Read the model definition and answer for the solid it produces. Units are mm, in the model's axes. Face numbers are marked on the shaded views. A direction names the side the tool comes from. Coordinates: 2 decimals unless noted, no trailing zeros. Loops run counter-clockwise (first coordinate to the right, second up) from the corner with the lowest first, then second, coordinate; pieces in that order, holes last. Notation, with made-up numbers: M -9,41 L 29,41 A16 ccw 29,65 Z; hole C 18,86.5 d2. An arc over 180 degrees is marked long. Use one line per item in the form item = value. Start each with the question number.
1. The part is cut by section A-A (x = 20.5). Give the vertices of the cut face in (y, z), plus the area to 3 significant figures.
2. The part is cut by section C-C (z = 12.5). Give the vertices of the cut face in (x, y).
3. A tool of negligible diameter and unlimited length cuts with its end or side. For the marked faces 4, 5 and 6, from which of +Z, -Z, +X, -X, +Y, -Y can it reach the whole face along a straight path? Write none if from no direction.
4. Flat-ended cylindrical pins translate along their axes: pin 1 (3 mm diameter, centred on y = 37, z = -24.5, fed in from +X); pin 2 (3 mm diameter, centred on x = 13.5, z = 20.5, fed in from +Y); pin 3 (12 mm diameter, centred on x = 12.5, z = 16, fed in from +Y); pin 4 (10 mm diameter, centred on y = -0.5, z = 29.5, fed in from -X). Find the tip coordinate at first contact, or state that the pin passes through.
5. For a pull along Y with two mould halves and no side action, classify the marked faces 1, 2 and 3 as released by +Y, released by -Y, zero draft, split by the parting line, or undercut.
6. The part is cut by section D-D (x = 28). Give the vertices of the cut face in (y, z), plus the area to 3 significant figures.
7. Find the intervals of material crossed by probe 1 along Y at (x, z) = (8, -8.5); probe 2 along Y at (x, z) = (28, 6); probe 3 along X at (y, z) = (-36, -13), in increasing order. Write a range as [from, to].
8. The part is cut by section B-B (y = 0). Give the vertices of the cut face in (x, z).
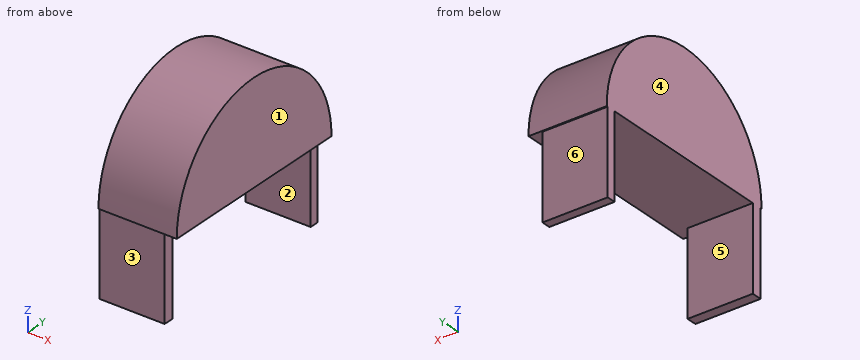
from build123d import *

# Parameters (mm, degrees)
F1_DEPTH = 5.08
F2_DEPTH = 25.4
F3_W     = 3.4888088703
F3_H     = 32.5622074306
F3_W_2   = 3.9539821446
F4_DEPTH = 25.4


with BuildPart() as f1:
    # F0 (on Right) → F1 (new body)
    with BuildSketch(Plane.YZ):
        with BuildLine():
            Line((-39.5398288965, 0), (39.5398288965, 0))
            ThreePointArc((39.5398288965, 0), (0, 39.5398288965), (-39.5398288965, 0))
        make_face()
    extrude(amount=F1_DEPTH)

    # F2 (add): a face of the model
    f2_faces = [f1.faces().sort_by_distance(p)[0] for p in [
        (5.08, 0, 16.781224581),
    ]]
    extrude(f2_faces, amount=F2_DEPTH)

    # F3 (on Right) → F4 (join)
    with BuildSketch(Plane.YZ):
        with Locations((37.3302474618, -16.2811037153)):
            Rectangle(F3_W, F3_H)
        with Locations((-37.0976608247, -16.2811037153)):
            Rectangle(F3_W_2, F3_H)
    extrude(amount=F4_DEPTH)


solid = f1.part
Computed values:
q1.outline = M -39.54,0 L -39.07,0 L -39.07,-32.56 L -35.12,-32.56 L -35.12,0 L 35.59,0 L 35.59,-32.56 L 39.07,-32.56 L 39.07,0 L 39.54,0 A39.54 ccw Z
q1.area = 2,700 mm²
q2.outline = M 0,-37.51 L 30.48,-37.51 L 30.48,37.51 L 0,37.51 Z
q3.face_4 = +Z, -Z, -X, +Y, -Y
q3.face_5 = -Z, +X, -X
q3.face_6 = -Z, +X, -X, +Y
q4.pin_1 = 25.4
q4.pin_2 = 34.68
q4.pin_3 = 38.25
q4.pin_4 = 0
q5.face_1 = zero draft
q5.face_2 = undercut
q5.face_3 = released by -Y
q6.outline = M -39.54,0 L 39.54,0 A39.54 ccw Z
q6.area = 2,460 mm²
q7.probe_1 = [-39.07, -35.12], [35.59, 39.07]
q7.probe_2 = [-39.08, 39.08]
q7.probe_3 = [0, 25.4]
q8.outline = M 0,0 L 30.48,0 L 30.48,39.54 L 0,39.54 Z
